```python
from build123d import *

# Parameters (mm, degrees)
SKETCH1_R           = 2.5
BOSS_EXTRUDE1_DEPTH = 42
SKETCH2_W           = 8.231649798
SKETCH2_H           = 2.477236303
CUT_EXTRUDE1_DEPTH  = 18
FILLET1_R           = 0.3


with BuildPart() as part:
    # Sketch1 → Boss-Extrude1 (new body)
    with BuildSketch(Plane(origin=(0, 0, 0), x_dir=(1, 0, 0), z_dir=(0, 1, 0))):
        with Locations(Location((0, 0, 0), (0, 0, 90))):
            Circle(SKETCH1_R)
    extrude(amount=BOSS_EXTRUDE1_DEPTH)

    # Sketch2 → Cut-Extrude1 (cut)
    with BuildSketch(Plane(origin=(0, 42, 0), x_dir=(1, 0, 0), z_dir=(0, 1, 0))):
        with Locations((-0.064511362, 3.238618152)):
            Rectangle(SKETCH2_W, SKETCH2_H)
    extrude(amount=-CUT_EXTRUDE1_DEPTH, mode=Mode.SUBTRACT)

    # Fillet1
    fillet1_edges = [part.edges().sort_by_distance(p)[0] for p in [
        (0, 42, 2.5),
    ]]
    fillet(fillet1_edges, radius=FILLET1_R)


solid = part.part
```
Source: CAD feature listing. Evaluate the final solid. Frame: model axes, mm. Coordinates: 2 decimals unless noted, no trailing zeros. Loops run counter-clockwise (first coordinate to the right, second up) from the corner with the lowest first, then second, coordinate; pieces in that order, holes last. Notation, with made-up numbers: (23, 39) -> (41, 39) arc R37 cw to (41, 75) -> close; hole circle Ø3 at (-39.5, 75.25). An arc over 180 degrees is marked (long way). One line per item, written item: value. Start each with the question number.
Q1. Section query A-A, the plane x = 0. Return the cut outline in (y, z).
Q2. Section query C-C, the plane y = 10. Return the cut outline in (x, z), and give its area (3 significant figures).
Q3. Line query: line 1 along Z through (x, y) = (0.2, 7); line 2 along Y through (x, z) = (2, -1); line 3 along X through (y, z) = (29.5, 2). Output: solid intervals per line, ascending.
Q4. Mould query, pull axis X, two halves, no side actions, for faces 1 (the face through (0, 33, -2)), 2 (the face through (-0.1, 20.6, 2.5)). Classes: pulls with the +X half, pulls with the -X half, needs draft (parallel to the pull), parting line crosses it, or undercut.
Q5. Section query B-B, the plane y = 32. Return the cut outline in (x, z).
Q6. Contact query for flat-ended pins moving along their axis: P1, Ø1.5, axis at x = -1.5, y = 28, coming from the +Z side; P2, Ø1.5, axis at x = 0.5, y = 33.5, coming from the -Z side. Output: stop coordinate, or through.
Results:
1. outline: (0, -2.5) -> (24, -2.5) -> (24, -2) -> (42, -2) -> (42, 2.2) arc R0.3 ccw to (41.7, 2.5) -> (0, 2.5) -> close
2. outline: circle Ø5 at (0, 0)
2. area: 19.6 mm^2
3. line 1: -2.49 to 2.49
3. line 2: 0 to 42
3. line 3: -1.5 to 1.5
4. face 1: needs draft
4. face 2: parting line crosses it
5. outline: (-1.5, -2) -> (1.5, -2) arc R2.5 ccw (long way) to start
6. P1: z = 2.38
6. P2: z = -2
